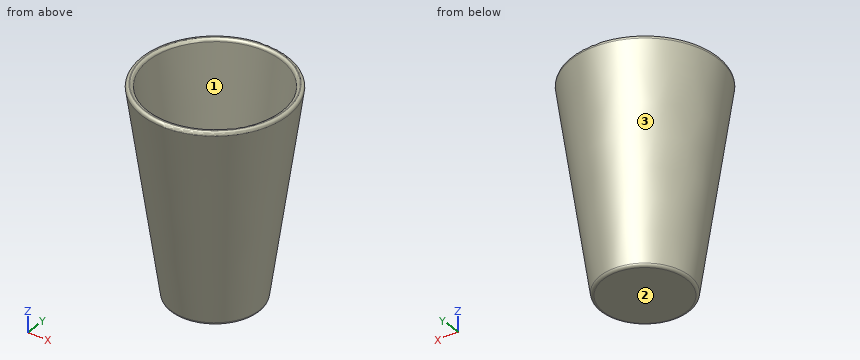
from build123d import *

# Parameters (mm, degrees)
FILLET_R = 1


with BuildPart() as cone001:
    # Cone001 → Cone001 (revolve)
    with BuildSketch(Plane(origin=(0, 0, 2), x_dir=(1, 0, 0), z_dir=(0, -1, 0))):
        Polygon((0, 0), (13, 0), (23, 70), (0, 70), align=None)
    revolve(axis=Axis((0, 0, 2), (0, 0, 1)))


with BuildPart() as fillet_body:
    # Cone → Cone (revolve)
    with BuildSketch(Plane.XZ):
        Polygon((0, 0), (15, 0), (25, 70), (0, 70), align=None)
    revolve(axis=Axis((0, 0, 0), (0, 0, 1)))

    # Cut: cut Cone001
    add(cone001.part, mode=Mode.SUBTRACT)

    # Fillet
    fillet_edges = [fillet_body.edges().sort_by_distance(p)[0] for p in [
        (-25, 0, 70),
        (-15, 0, 0),
        (-22.714286, 0, 70),
        (-13, 0, 2),
    ]]
    fillet(fillet_edges, radius=FILLET_R)


solid = fillet_body.part
The model under review builds one solid part; all positions refer to its coordinate system, in mm. Face numbers are marked on the shaded views. Round coordinates to 2 decimals unless told otherwise and drop trailing zeros. Order: outer loops, then holes, each group sorted by start corner. A loop starts at its lowest first (then second) coordinate and runs counter-clockwise, first axis right, second up. Notation, with made-up numbers: (16.5, -35) - (60.5, -35) arc R19 cw to (60.5, -16) - close; hole circle Ø3 at (35.5, 29). An arc over 180 degrees is marked (long way). Use one line per item in the form item = value.
Q1. Add section C-C on z = 35.5. Give the boundary of the cut face in (x, y).
Response values:
outline = circle Ø40.14 at (0, 0); hole circle Ø35.57 at (0, 0)
Q2. Clearance check with flat-ended pins moving along their axes: P1, Ø1.5, axis at y = 9.5, z = 31, coming from the -X side; P2, Ø10, axis at y = 13.5, z = 24.5, coming from the +X side; P3, Ø6, axis at y = -18, z = 38, coming from the +X side. State where each tip first meets the part, or that it passes through.
Response values:
P1 = -17.37
P2 = 16.55
P3 = 13.93
Q3. Add section D-D on z = 7. Give the boundary of the cut face in (x, y).
Response values:
outline = circle Ø32 at (0, 0); hole circle Ø27.43 at (0, 0)
Q4. To check wall thickness, follow line 1 (Z direction, x = -7, y = 5); line 2 (X direction, y = 13, z = 28); line 3 (X direction, y = -2.5, z = 27.5). State the ranges of each line that lie inside material, in increasing order.
Response values:
line_1 = 0 to 2
line_2 = -13.86 to -10.51, 10.51 to 13.86
line_3 = -18.76 to -16.45, 16.45 to 18.76
Q5. Mouldability with a two-part tool opening along X and no side actions: class the marked faces 1, 2 and 3 as pulls with the +X half, pulls with the -X half, needs draft (parallel to the pull), parting line crosses it, or undercut.
Response values:
face_1 = undercut
face_2 = needs draft
face_3 = parting line crosses it
Q6. Add section A-A on y = 0. Give the boundary of the cut face in (x, z).
Response values:
outline = (-24.84, 68.86) - (-15.12, 0.86) arc R1 ccw to (-14.13, 0) - (14.13, 0) arc R1 ccw to (15.12, 0.86) - (24.84, 68.86) arc R1 ccw to (23.85, 70) - (23.58, 70) arc R1 ccw to (22.59, 69.14) - (13.12, 2.86) arc R1 cw to (12.13, 2) - (-12.13, 2) arc R1 cw to (-13.12, 2.86) - (-22.59, 69.14) arc R1 ccw to (-23.58, 70) - (-23.85, 70) arc R1 ccw to start
